from build123d import *

# Parameters (mm, degrees)
F1_DEPTH = 127
F2_R     = 113.665
F2_R_2   = 69.85
F3_DEPTH = 76.2
F2_R_3   = 34.798
F4_DEPTH = 101.6


with BuildPart() as f1:
    # F0 (on Front) → F1 (new body, symmetric)
    with BuildSketch(Plane.XZ):
        Polygon((127, 0), (0, 0), (0, -30.48), (96.52, -30.48), (96.52, -85.344), (127, -85.344), align=None)
        Polygon((0, -30.48), (0, 0), (-127, 0), (-127, -85.344), (-96.52, -85.344), (-96.52, -30.48), align=None)
    extrude(amount=F1_DEPTH, both=True)

    # F2 (on face) → F3 (join)
    with BuildSketch(Plane.XY):
        Circle(F2_R)
        Circle(F2_R_2, mode=Mode.SUBTRACT)
    extrude(amount=F3_DEPTH)

    # F2 (on face) → F4 (cut)
    with BuildSketch(Plane.XY):
        Circle(F2_R_3)
    extrude(amount=-F4_DEPTH, mode=Mode.SUBTRACT)


solid = f1.part
Geometry: final body of the model. Coordinates: model frame, mm. A direction names the side the tool comes from. Give positions to 0.01 mm unless a question says otherwise; leave off trailing zeros. Write each loop counter-clockwise with the first axis right and the second up, starting at its lowest first coordinate (ties: lowest second). Pieces come first, ordered by that corner, then holes. Notation, with made-up numbers: (-4, 6.5) -> (49, 6.5) arc R6 cw to (49, 13.5) -> close; hole circle Ø4 at (12.5, -9). An arc over 180 degrees is marked (long way). Answer as a JSON object with one key per item and string values.
1. Mould query, pull axis X, two halves, no side actions, for faces 4 (the flat face through (115, -2, 0)), 5 (the cylindrical face through (52.45, -100.84, 37.57)), 6 (the flat face through (96.52, -2, -58)). Classes: pulls with the +X half, pulls with the -X half, needs draft (parallel to the pull), parting line crosses it, or undercut.
Ans:
{"face 4": "needs draft", "face 5": "parting line crosses it", "face 6": "undercut"}
2. Access query for faces 1 (the flat face through (-2, 127, -23)), 2 (the cylindrical face through (-55.431, -42.503, 37.567)), 3 (the flat face through (-23, -30, -30.48)). Directions: +Z, -Z, +X, -X, +Y, -Y. A direction counts if a zero-diameter tool reaches every point of the face in a straight line with its end or side. Return the directions, or none.
Ans:
{"face 1": "+Z, -Z, +X, -X, +Y", "face 2": "+Z", "face 3": "-Z, +Y, -Y"}
3. Contact query for flat-ended pins moving along their axis: pin 1 (3 mm diameter, centred on x = 3, z = 50.5, fed in from -Y); pin 2 (8 mm diameter, centred on y = 90.5, z = 27.5, fed in from -X); pin 3 (5 mm diameter, centred on x = 42.5, y = -55, fed in from +Z); pin 4 (2 mm diameter, centred on x = -12, y = -88, fed in from -Z). Output: stop coordinate, or through.
Ans:
{"pin 1": "stops at y = -113.66", "pin 2": "stops at x = -73.74", "pin 3": "stops at z = 76.2", "pin 4": "stops at z = -30.48"}
4. Cut plane A-A on x = 0. Output: boundary loops of the cut face in (y, z) (3 decimals), and give its area (3 significant figures).
Ans:
{"outline": "(-127, -30.48) -> (-34.798, -30.48) -> (-34.798, 0) -> (-69.85, 0) -> (-69.85, 76.2) -> (-113.665, 76.2) -> (-113.665, 0) -> (-127, 0) -> close; (34.798, -30.48) -> (127, -30.48) -> (127, 0) -> (113.665, 0) -> (113.665, 76.2) -> (69.85, 76.2) -> (69.85, 0) -> (34.798, 0) -> close", "area": "12,300 mm^2"}
5. Cut plane D-D on x = 66. Output: boundary loops of the cut face in (y, z).
Ans:
{"outline": "(-127, -30.48) -> (127, -30.48) -> (127, 0) -> (92.54, 0) -> (92.54, 76.2) -> (22.87, 76.2) -> (22.87, 0) -> (-22.87, 0) -> (-22.87, 76.2) -> (-92.54, 76.2) -> (-92.54, 0) -> (-127, 0) -> close"}
6. Cut plane B-B on y = 0. Output: boundary loops of the cut face in (x, z) (3 decimals), and give its area (3 significant figures).
Ans:
{"outline": "(-127, -85.344) -> (-96.52, -85.344) -> (-96.52, -30.48) -> (-34.798, -30.48) -> (-34.798, 0) -> (-69.85, 0) -> (-69.85, 76.2) -> (-113.665, 76.2) -> (-113.665, 0) -> (-127, 0) -> close; (34.798, -30.48) -> (96.52, -30.48) -> (96.52, -85.344) -> (127, -85.344) -> (127, 0) -> (113.665, 0) -> (113.665, 76.2) -> (69.85, 76.2) -> (69.85, 0) -> (34.798, 0) -> close", "area": "15,600 mm^2"}
7. Ray query, probe 1 along X at (y, z) = (62, -54.5); probe 2 along Y at (x, z) = (0, 59.5) (3 decimals); probe 3 along Y at (x, z) = (0, -10). Return the intervals inside material, ascending. Write a range as from..to.
Ans:
{"probe 1": "x = -127..-96.52, 96.52..127", "probe 2": "y = -113.665..-69.85, 69.85..113.665", "probe 3": "y = -127..-34.8, 34.8..127"}
8. Cut plane C-C on z = 6.5. Output: boundary loops of the cut face in (x, y) (3 decimals).
Ans:
{"outline": "circle Ø227.33 at (0, 0); hole circle Ø139.7 at (0, 0)"}
